Build history of the part. All positions in model axes, mm. A direction names the side the tool comes from. Give positions to 0.01 mm unless a question says otherwise; leave off trailing zeros. Write each loop counter-clockwise with the first axis right and the second up, starting at its lowest first coordinate (ties: lowest second). Pieces come first, ordered by that corner, then holes. Notation, with made-up numbers: (32, 70.5) -> (62, 70.5) arc R26 ccw to (62, 107.5) -> close; hole circle Ø2 at (76, 80). An arc over 180 degrees is marked (long way). Put each result on its own line as item: value.
from build123d import *

# Parameters (mm, degrees)
F0_W     = 114.3
F0_H     = 4.5211492
F0_H_2   = 17.9908454
F1_DEPTH = 5.08
F2_DEPTH = 15.494
F3_START = 15.494
F3_DEPTH = 4.826


with BuildPart() as f1:
    # F0 (on Top) → F1 (new body)
    with BuildSketch(Plane.XY):
        with Locations((5.5734652638, -23.0715045245)):
            Rectangle(F0_W, F0_H)
        with Locations((5.5734652638, -34.3275018245)):
            Rectangle(F0_W, F0_H_2)
    extrude(amount=-F1_DEPTH)

    # F0 (on Top) → F2 (join)
    with BuildSketch(Plane.XY):
        with Locations((5.5734652638, -34.3275018245)):
            Rectangle(F0_W, F0_H_2)
    extrude(amount=F2_DEPTH)

    # F0 (on Top) → F3 (join)
    with BuildSketch(Plane.XY.offset(F3_START)):
        with Locations((5.5734652638, -23.0715045245)):
            Rectangle(F0_W, F0_H)
        with Locations((5.5734652638, -34.3275018245)):
            Rectangle(F0_W, F0_H_2)
    extrude(amount=F3_DEPTH)


solid = f1.part
1) Tool access for faces 1 (the flat face through (5, -23, 0)), 2 (the flat face through (5, -20.811, -3)): list every direction of +Z, -Z, +X, -X, +Y, -Y with a clear straight run to the whole face (end or side of a thin tool).
Filled sheet:
face 1: +X, -X, +Y
face 2: +Z, -Z, +X, -X, +Y
2) Slice it at A-A (y = -22.5). Write the cut outline in (x, z).
Filled sheet:
outline: (-51.58, -5.08) -> (62.72, -5.08) -> (62.72, 0) -> (-51.58, 0) -> close; (-51.58, 15.49) -> (62.72, 15.49) -> (62.72, 20.32) -> (-51.58, 20.32) -> close
3) Slice it at C-C (z = 4.25). Write the cut outline in (x, y).
Filled sheet:
outline: (-51.58, -43.32) -> (62.72, -43.32) -> (62.72, -25.33) -> (-51.58, -25.33) -> close
4) Pull direction Z, two halves, no side cores. Call faces 3 (the flat face through (5, -32, 20.32)), 4 (the flat face through (5, -23, 15.494)), 5 (the flat face through (62.723, -32, 7)): released by +Z, released by -Z, zero draft, split by the parting line, or undercut.
Filled sheet:
face 3: released by +Z
face 4: undercut
face 5: zero draft
5) Wall check: L1, parallel to Z at x = 2.5, y = -24.25; L2, parallel to Y at x = -36, z = 14.75. Give the ranges that are in metal, low to high.
Filled sheet:
L1: -5.08 to 0, 15.49 to 20.32
L2: -43.32 to -25.33
6) Slice it at B-B (x = 41.5). Write the cut outline in (y, z).
Filled sheet:
outline: (-43.32, -5.08) -> (-20.81, -5.08) -> (-20.81, 0) -> (-25.33, 0) -> (-25.33, 15.49) -> (-20.81, 15.49) -> (-20.81, 20.32) -> (-43.32, 20.32) -> close
